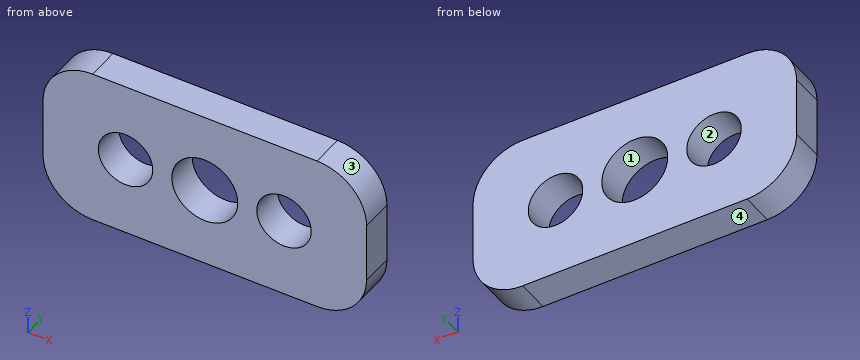
from build123d import *

# Parameters (mm, degrees)
F0_W     = 19.6
F0_H     = 9.6
F1_DEPTH = 2
F2_R     = 2
F3_DEPTH = 3
F4_R     = 1.65
F6_DEPTH = 3
F5_R     = 1.65
F7_DEPTH = 3
F8_R     = 3


with BuildPart() as f1:
    # F0 (on Front) → F1 (new body)
    with BuildSketch(Plane.XZ):
        with Locations((9.8, 4.8)):
            Rectangle(F0_W, F0_H)
    extrude(amount=F1_DEPTH)

    # F2 (on face) → F3 (cut)
    with BuildSketch(Plane.XZ.offset(2)):
        with Locations((9.8, 4.8)):
            Circle(F2_R)
    extrude(amount=-F3_DEPTH, mode=Mode.SUBTRACT)

    # F4 (on face) → F6 (cut)
    with BuildSketch(Plane.XZ.offset(2)):
        with Locations((5, 4.8)):
            Circle(F4_R)
    extrude(amount=-F6_DEPTH, mode=Mode.SUBTRACT)

    # F5 (on face) → F7 (cut)
    with BuildSketch(Plane.XZ.offset(2)):
        with Locations((14.6, 4.8)):
            Circle(F5_R)
    extrude(amount=-F7_DEPTH, mode=Mode.SUBTRACT)

    # F8
    f8_edges = [f1.edges().sort_by_distance(p)[0] for p in [
        (19.6, -1, 9.6),
        (0, -1, 9.6),
        (0, -1, 0),
        (19.6, -1, 0),
    ]]
    fillet(f8_edges, radius=F8_R)


solid = f1.part
Geometry check sheet. Reference: the model listing, model coordinates, mm. Face numbers are marked on the shaded views. Give positions to 0.01 mm unless a question says otherwise; leave off trailing zeros. Loops run counter-clockwise (first coordinate to the right, second up) from the corner with the lowest first, then second, coordinate; pieces in that order, holes last.
(1) Section check C-C on y = -1.7. Record the cut outline in (x, z).
From the geometry:
outline: (0, 3) arc R3 ccw to (3, 0) - (16.6, 0) arc R3 ccw to (19.6, 3) - (19.6, 6.6) arc R3 ccw to (16.6, 9.6) - (3, 9.6) arc R3 ccw to (0, 6.6) - close; hole circle Ø3.3 at (5, 4.8); hole circle Ø4 at (9.8, 4.8); hole circle Ø3.3 at (14.6, 4.8)
(2) Section check D-D on x = 9.8. Record the cut outline in (y, z), then the cut area to 3 significant figures.
From the geometry:
outline: (-2, 0) - (0, 0) - (0, 2.8) - (-2, 2.8) - close; (-2, 6.8) - (0, 6.8) - (0, 9.6) - (-2, 9.6) - close
area: 11.2 mm2
(3) Section check A-A on x = 5. Record the cut outline in (y, z), then the cut area to 3 significant figures.
From the geometry:
outline: (-2, 0) - (0, 0) - (0, 3.15) - (-2, 3.15) - close; (-2, 6.45) - (0, 6.45) - (0, 9.6) - (-2, 9.6) - close
area: 12.6 mm2
(4) Release check for a two-part mould opening along X. For the marked faces 1, 2, 3 and 4 record: released by +X, released by -X, zero draft, split by the parting line, or undercut.
From the geometry:
face 1: undercut
face 2: undercut
face 3: released by +X
face 4: zero draft
(5) Thickness scan on L1, parallel to Z at x = 5, y = -1.1; L2, parallel to X at y = -0.6, z = 3.5; L3, parallel to X at y = -0.5, z = 6. Record the ranges inside material, lowest first.
From the geometry:
L1: z = 0 to 3.15, 6.45 to 9.6
L2: x = 0 to 3.98, 6.02 to 8.28, 11.32 to 13.58, 15.62 to 19.6
L3: x = 0 to 3.87, 6.13 to 8.2, 11.4 to 13.47, 15.73 to 19.6
(6) Section check B-B on z = 4.8. Record the cut outline in (x, y), then the cut area to 3 significant figures.
From the geometry:
outline: (0, -2) - (3.35, -2) - (3.35, 0) - (0, 0) - close; (6.65, -2) - (7.8, -2) - (7.8, 0) - (6.65, 0) - close; (11.8, -2) - (12.95, -2) - (12.95, 0) - (11.8, 0) - close; (16.25, -2) - (19.6, -2) - (19.6, 0) - (16.25, 0) - close
area: 18.0 mm2
(7) Depth check by flat-ended pin: pin 1 Ø2.5 at (x, z) = (5, 4.8) entering from -Y. Enter the tip coordinate at first touch or a pass-through.
From the geometry:
pin 1: passes through
